Here's how the part is built. I have some questions about the finished solid (model axes, mm). Give positions to 0.01 mm unless a question says otherwise; leave off trailing zeros. Loops run counter-clockwise (first coordinate to the right, second up) from the corner with the lowest first, then second, coordinate; pieces in that order, holes last. Notation, with made-up numbers: (17.25, -40) - (64.25, -40) arc R16 cw to (64.25, -31) - close; hole circle Ø3 at (60.5, 38.25). An arc over 180 degrees is marked (long way). Return JSON: item names as keys, results as strings. Group by question number.
(1) For P1, Ø5, axis at x = 8, y = 84.5, coming from the -Z side; P2, Ø6, axis at x = -1, z = -9, coming from the -Y side; P3, Ø2, axis at x = 2, z = -10, coming from the -Y side, each with a flat end and sliding along its axis, tell me the tip position at first contact or that it passes through.
(2) If we section it at C-C (x = -8.75): Please give me the cut outline in (y, z).
(3) If we section it at A-A (z = -6.75): Please give me the cut outline in (x, y).
(4) If we section it at B-B (y = 126): Please give me the cut outline in (x, z).
(5) I need wall thicknesses on probe 1 along Z at (x, y) = (3, 125); probe 2 along Y at (x, z) = (-2.5, -16); probe 3 along Y at (x, z) = (1, -7.5). Which ranges of each line are inside material? Lowest first, please. Write a range as [from, to].
(6) If we section it at D-D (z = -15.75): Please give me the cut outline in (x, y).
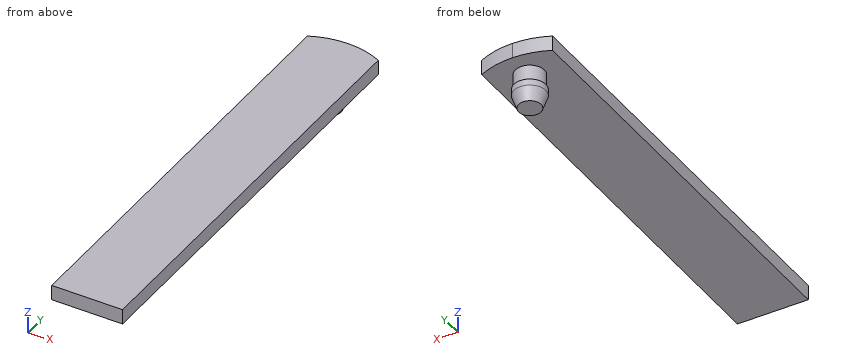
```python
from build123d import *

# Parameters (mm, degrees)
F1_DEPTH = 5.2
F2_R     = 5
F3_DEPTH = 5.4
F5_R     = 5.5
F6_DEPTH = 2.2
F10_R    = 5.5
F8_R     = 3.85


with BuildPart() as f1:
    # F0 (on Top) → F1 (new body)
    with BuildSketch(Plane.XY):
        Polygon((-12.2, 0), (0, 0), (12.2, 0), (12.2, 148.6), (0, 148.6), (-12.2, 148.6), align=None)
        with BuildLine():
            Line((0, 148.6), (12.2, 148.6))
            ThreePointArc((12.2, 148.6), (6.2585940913, 150.6910171122), (0, 151.4))
            Line((0, 151.4), (0, 148.6))
        make_face()
        with BuildLine():
            ThreePointArc((0, 151.4), (-6.2585940913, 150.6910171122), (-12.2, 148.6))
            Line((-12.2, 148.6), (0, 148.6))
            Line((0, 148.6), (0, 151.4))
        make_face()
    extrude(amount=-F1_DEPTH)

    # F2 (on face) → F3 (join)
    with BuildSketch(Plane(origin=(0, 0, -5.2), x_dir=(1, 0, 0), z_dir=(0, 0, -1))):
        with Locations((0, -141.2)):
            Circle(F2_R)
    extrude(amount=F3_DEPTH)

    # F5 (on offset) → F6 (join)
    with BuildSketch(Plane(origin=(0, 0, -10.6), x_dir=(1, 0, 0), z_dir=(0, 0, -1))):
        with Locations((0, -141.2)):
            Circle(F5_R)
    extrude(amount=F6_DEPTH)

    # F10 (on offset) → F11 section 0
    with BuildSketch(Plane(origin=(0, 0, -12.8), x_dir=(1, 0, 0), z_dir=(0, 0, -1))):
        with Locations((0, -141.2)):
            Circle(F10_R)
    # F8 (on offset) → F11 section 1
    with BuildSketch(Plane(origin=(0, 0, -17.3), x_dir=(1, 0, 0), z_dir=(0, 0, -1))):
        with Locations((0, -141.2)):
            Circle(F8_R)
    loft()


solid = f1.part
```
Values:
{
 "1": {"P1": "z = -5.2", "P2": "y = 135.7", "P3": "y = 135.83"},
 "2": {"outline": "(0, -5.2) - (150, -5.2) - (150, 0) - (0, 0) - close"},
 "3": {"outline": "circle Ø10 at (0, 141.2)"},
 "4": {"outline": "(-12.2, -5.2) - (12.2, -5.2) - (12.2, 0) - (-12.2, 0) - close"},
 "5": {"probe 1": "[-5.2, 0]", "probe 2": "[137.67, 144.73]", "probe 3": "[136.3, 146.1]"},
 "6": {"outline": "circle Ø8.84 at (0, 141.2)"}
}
